Can you work these out from the model? Positions are in its coordinate system, mm. A direction names the side the tool comes from. Give positions to 0.01 mm unless a question says otherwise; leave off trailing zeros. Order: outer loops, then holes, each group sorted by start corner. A loop starts at its lowest first (then second) coordinate and runs counter-clockwise, first axis right, second up. Notation, with made-up numbers: (-28, 1.5) - (-10, 1.5) arc R30 cw to (-10, 34.5) - close; hole circle Ø9 at (83, -2). An arc over 180 degrees is marked (long way). Return JSON: item names as keys, results as strings.
Autodesk Inventor part; units mm, degrees
ref_plane "Arbeitsebene1" through (0, 0, 0) normal (1, 0, 0) x (0, 1, 0)
ref_plane "XZ Plane" through (0, 0, 0) normal (0, 1, 0) x (-1, 0, 0)
ref_plane "XY Plane" through (0, 0, 0) normal (0, 0, 1) x (1, 0, 0)
sketch "Skizze2" plane through (0, 0, 0) normal (0, 0, 1) x (1, 0, 0)
  circle A0 centre (0, 0) radius 50
  circle A1 centre (0, 0) radius 41.5 construction
  dimension "d12" = 100
  dimension "d13" = 83
extrude "Extrusion3" add sketch "Skizze2" against normal blind 10
sketch "Skizze3" plane through (0, 0, 0) normal (0, 0, 1) x (1, 0, 0)
  circle A0 centre (0, 0) radius 50
  line L0 (0, 50) -> (0, -50) construction
  line L1 (-50, 0) -> (50, 0) construction
  line L2 (0, -10) -> (-13.0826, -39.384)
  line L3 (0, -10) -> (13.0826, -39.384)
  circle A1 centre (0, 0) radius 41.5 construction
  arc A2 (-13.0826, -39.384) -> (13.0826, -39.384) centre (0, 0) ccw
  dimension "d16" = 48
  dimension "d17" = 10
extrude "Extrusion4" cut sketch "Skizze3" against normal up to surface (10 mm away) contours L3 A2 L2
pattern_circular "Runde Anordnung1" count 2 over 360 about axis through (0, 0, 0) along (0, 0, -1) of "Extrusion4"
sketch "Skizze4" plane through (0, 0, 0) normal (0, 0, 1) x (1, 0, 0)
  line L0 (-50, 0) -> (50, 0) construction
  line L1 (0, 50) -> (0, -50) construction
  line L2 (-3.6024, 1.25) -> (3.6024, 1.25)
  line L3 (-3.6024, -1.25) -> (3.6024, -1.25)
  line L4 (3.6024, 1.25) -> (25.0677, 33.0736)
  circle A0 centre (0, 0) radius 41.5 construction
  line L5 (13.0826, 39.384) -> (0, 10)
  line L6 (3.6024, -1.25) -> (11.6965, -13.25)
  line L7 (11.6965, -13.25) -> (35.325, 21.7807)
  line L8 (0, -10) -> (13.0826, -39.384)
  arc A1 (35.325, 21.7807) -> (25.0677, 33.0736) centre (0, 0) ccw
  line L9 (-3.6024, 1.25) -> (-25.0677, 33.0736)
  line L10 (0, 10) -> (-13.0826, 39.384)
  line L11 (-3.6024, -1.25) -> (-11.6965, -13.25)
  line L12 (-11.6965, -13.25) -> (-35.325, 21.7807)
  arc A2 (-25.0677, 33.0736) -> (-35.325, 21.7807) centre (0, 0) ccw
  line L13 (-13.0826, -39.384) -> (0, -10)
  dimension "d23" = 2.5
  dimension "d30" = 12
  dimension "d31" = 10
  dimension "d32" = 10
  dimension "d33" = 10
  dimension "d34" = 10
extrude "Extrusion5" cut sketch "Skizze4" against normal up to surface (10 mm away)
sketch "Skizze5" plane through (0, 0, 0) normal (0, 0, 1) x (1, 0, 0)
  circle A0 centre (0, 0) radius 41.5 construction
  line L0 (0, 50) -> (0, -50) construction
  line L1 (-50, 0) -> (50, 0) construction
  line L2 (-11.6965, -13.25) -> (-35.325, 21.7807)
  line L3 (-41.352, 3.5016) -> (-25.0677, -33.0736)
  line L4 (-13.4789, -15.8926) -> (-28.8614, -38.698) construction
  line L5 (-3.6024, -1.25) -> (-11.6965, -13.25)
  arc A1 (-41.352, 3.5016) -> (-25.0677, -33.0736) centre (0, 0) ccw
  point P0 (-33.2098, -14.786)
  dimension "d41" = 10
extrude "Extrusion6" cut sketch "Skizze5" against normal up to surface (10 mm away)
ref_plane "Arbeitsebene1" through (0, 0, 0) normal (1, 0, 0) x (0, 1, 0)
mirror "Spiegeln1" about plane through (0, 0, 0) normal (1, 0, 0) of "Extrusion6"
equation "\"d32\" = d31"
properties part number "VW" material "Stahl, galvanisiert"
1. If I drill on L1, parallel to X at y = 4, z = -5.25; L2, parallel to Y at x = 26.5, z = -1.5; L3, parallel to Y at x = 31, z = -9, over which ranges is the centre line in solid material (lowest first)? Write a range as [from, to].
Checks:
{"L1": "[-49.84, -23.33], [-5.46, 5.46], [23.33, 49.84]", "L2": "[-42.4, -31.94], [-29.86, 8.7], [31.94, 42.4]", "L3": "[-39.23, -27.59], [-19.75, 15.37], [27.59, 39.23]"}
2. Suppose I cut it at B-B (y = -20). List the corners of the cut face in (x, z) for me, plus the area to 3 significant figures.
Checks:
{"outline": "(-45.83, -10) - (-36.36, -10) - (-36.36, 0) - (-45.83, 0) - close; (-30.89, -10) - (-4.45, -10) - (-4.45, 0) - (-30.89, 0) - close; (4.45, -10) - (30.89, -10) - (30.89, 0) - (4.45, 0) - close; (36.36, -10) - (45.83, -10) - (45.83, 0) - (36.36, 0) - close", "area": "718 mm^2"}
3. Suppose I cut it at C-C (x = 40). List the corners of the cut face in (y, z) for me.
Checks:
{"outline": "(-30, -10) - (-11.06, -10) - (-11.06, 0) - (-30, 0) - close; (0.46, -10) - (30, -10) - (30, 0) - (0.46, 0) - close"}
4. Thinking about a two-plate mould opening in Y: for faces 3 (the face through (-1, -10, -10)), 4 (the face through (47.69, 15.02, -4.93)), 5 (the face through (23.345, 4.02, -4.93)), which applies, +Y half, -Y half, draft (parallel to the pull), parting line (faces both ways), or undercut?
Checks:
{"face 3": "draft", "face 4": "parting line", "face 5": "undercut"}
5. Suppose I cut it at A-A (z = -1.25). State how many separate pieces and enclosed holes the cut face has, plus the area to 3 significant figures.
Checks:
{"separate pieces": "1", "enclosed holes": "5", "area": "5,480 mm^2"}
6. Suppose I cut it at D-D (y = 37.5). List the corners of the cut face in (x, z) for me.
Checks:
{"outline": "(-33.07, -10) - (-12.24, -10) - (-12.24, 0) - (-33.07, 0) - close; (12.24, -10) - (33.07, -10) - (33.07, 0) - (12.24, 0) - close"}
7. On a 3-axis mill with a long thin cutter (end or side, diameter ignored), from which of +Z, -Z, +X, -X, +Y, -Y can I reach the whole of each face in a straight line? I mean faces 1 (the face through (33.096, -15.042, -4.93)), 2 (the face through (-1, -10, 0)). Say none if no direction works.
Checks:
{"face 1": "+Z, -Z", "face 2": "+Z, +X, -X, +Y, -Y"}
8. For pin 1 Ø3.5 at (x, z) = (1.5, -6.5) entering from +Y; pin 2 Ø3.5 at (x, z) = (0, -5.5) entering from -Y; pin 3 Ø1 at (x, z) = (10, -8) entering from +Y; pin 4 Ø4 at (x, y) = (35.5, -17) entering from -Z, each with a flat end and sliding along its axis, tell me the tip position at first contact or that it passes through.
Checks:
{"pin 1": "y = 50", "pin 2": "y = -50", "pin 3": "y = 49.09", "pin 4": "through"}
